Verification items for the finished model (mm, model axes). A direction names the side the tool comes from. Coordinates: 2 decimals unless noted, no trailing zeros. Write each loop counter-clockwise with the first axis right and the second up, starting at its lowest first coordinate (ties: lowest second). Pieces come first, ordered by that corner, then holes.
```python
from build123d import *

# Parameters (mm, degrees)
F0_W          = 30
F0_H          = 30
F1_DEPTH      = 865
F2_W          = 30
F2_H          = 30
F3_DEPTH      = 257.5
F3_DEPTH_BACK = 257.5
F4_W          = 30
F4_H          = 30
F5_DEPTH      = 215
F5_DEPTH_BACK = 215
F6_W          = 480
F6_H          = 30
F7_DEPTH      = 1.5
F8_W          = 480
F8_H          = 1.5
F9_DEPTH      = 28.5
F10_R         = 5


with BuildPart() as f1:
    # F0 (on Top) → F1 (new body)
    with BuildSketch(Plane.XY):
        with Locations((-272.5, 230)):
            Rectangle(F0_W, F0_H)
        with Locations((272.5, 230)):
            Rectangle(F0_W, F0_H)
        with Locations((272.5, -230)):
            Rectangle(F0_W, F0_H)
        with Locations((-272.5, -230)):
            Rectangle(F0_W, F0_H)
    extrude(amount=F1_DEPTH)

    # F2 (on Right) → F3 (join, two sides)
    with BuildSketch(Plane.YZ) as f3_sk:
        with Locations((-230, 100)):
            Rectangle(F2_W, F2_H)
        with Locations((230, 100)):
            Rectangle(F2_W, F2_H)
        with Locations((-230, 850)):
            Rectangle(F2_W, F2_H)
        with Locations((230, 850)):
            Rectangle(F2_W, F2_H)
    extrude(amount=F3_DEPTH)
    extrude(f3_sk.sketch, amount=-F3_DEPTH_BACK)

    # F4 (on Front) → F5 (join, two sides)
    with BuildSketch(Plane.XZ) as f5_sk:
        with Locations((-272.5, 850)):
            Rectangle(F4_W, F4_H)
        with Locations((272.5, 850)):
            Rectangle(F4_W, F4_H)
    extrude(amount=F5_DEPTH)
    extrude(f5_sk.sketch, amount=-F5_DEPTH_BACK)



with BuildPart() as f7:
    # F6 (on face) → F7 (new body)
    with BuildSketch(Plane.YZ.offset(-257.5)):
        with Locations((0, 130)):
            Rectangle(F6_W, F6_H)
        with Locations((0, 300)):
            Rectangle(F6_W, F6_H)
        with Locations((0, 470)):
            Rectangle(F6_W, F6_H)
        with Locations((0, 640)):
            Rectangle(F6_W, F6_H)
    extrude(amount=F7_DEPTH)


with BuildPart() as f1_1:
    add(f1.part)

    add(f7.part)  # F9 merges F7
    # F8 (on face) → F9 (join)
    with BuildSketch(Plane.YZ.offset(-256)):
        with Locations((0, 115.75)):
            Rectangle(F8_W, F8_H)
        with Locations((0, 285.75)):
            Rectangle(F8_W, F8_H)
        with Locations((0, 455.75)):
            Rectangle(F8_W, F8_H)
        with Locations((0, 625.75)):
            Rectangle(F8_W, F8_H)
    extrude(amount=F9_DEPTH)

    # F10
    f10_edges = [f1_1.edges().sort_by_distance(p)[0] for p in [
        (-256.75, -240, 145),
        (-256.75, 240, 145),
        (-227.5, 240, 115.75),
        (-227.5, -240, 115.75),
        (-256.75, -240, 315),
        (-227.5, -240, 285.75),
        (-227.5, -240, 455.75),
        (-256.75, -240, 485),
        (-227.5, -240, 625.75),
        (-256.75, -240, 655),
        (-256.75, 240, 655),
        (-227.5, 240, 625.75),
        (-227.5, 240, 455.75),
        (-256.75, 240, 485),
        (-227.5, 240, 285.75),
        (-256.75, 240, 315),
    ]]
    fillet(f10_edges, radius=F10_R)

    # F11: F1 across plane


with BuildPart() as f1_2:
    add(f1_1.part)
    add(f1_1.part.mirror(Plane.YZ))


solid = f1_2.part
```
1. Material ranges on L1, parallel to Z at x = -253.5, y = 135.5; L2, parallel to Z at x = -235.5, y = -224; L3, parallel to X at y = 211, z = 633.5, recorded low to high.
2. Tool access check on faces 4 (the flat face through (272, -3, 835)), 5 (the flat face through (-251, -240, 286)), 6 (the flat face through (-257.5, -3, 300)), 7 (the flat face through (-257.5, 230, 42)), 8 (the flat face through (-256, -3, 471)). Record the directions out of +Z, -Z, +X, -X, +Y, -Y that give a thin tool (end or side, any length) a straight path to the whole face; none if there is none.
3. Sectioned sample at A-A, the plane x = -62. Record the boundary of the cut face in (y, z), and give its area (3 significant figures).
4. Gauge pin test, flat ends, axial feed: P1, Ø14, axis at y = -6.5, z = 133.5, coming from the +X side; P2, Ø1.6, axis at x = 256.5, y = -40.5, coming from the +Z side; P3, Ø8.5, axis at x = -238.5, y = -100.5, coming from the +Z side; P4, Ø20, axis at x = 251, z = 464.5, coming from the -Y side. Record the tip position at first contact, or that the pin passes through.
5. Sectioned sample at C-C, the plane x = -244. Give the number of separate pieces and of enclosed holes in the cut face, and give its area (3 significant figures).
6. Sectioned sample at B-B, the plane z = 504. Record the boundary of the cut face in (x, y).
7. Draft check along Z on faces 1 (the flat face through (-243, -3, 115)), 2 (the flat face through (-257.5, -230, 42)), 3 (the flat face through (-4, -230, 835)). Enter one of: pulls with the +Z half, pulls with the -Z half, needs draft (parallel to the pull), parting line crosses it, or undercut.
Outcome:
1. L1: z = 115 to 116.5, 285 to 286.5, 455 to 456.5, 625 to 626.5
1. L2: z = 85 to 116.5, 285 to 286.5, 455 to 456.5, 625 to 626.5, 835 to 865
1. L3: x = -257.5 to -256, 256 to 257.5
2. face 4: -Z, +X, -X
2. face 5: -Y
2. face 6: -Z, -X
2. face 7: -Z, +Y, -Y
2. face 8: +Y, -Y
3. outline: (-245, 85) - (-215, 85) - (-215, 115) - (-245, 115) - close; (-245, 835) - (-215, 835) - (-215, 865) - (-245, 865) - close; (215, 85) - (245, 85) - (245, 115) - (215, 115) - close; (215, 835) - (245, 835) - (245, 865) - (215, 865) - close
3. area: 3,600 mm2
4. P1: stops at x = 257.5
4. P2: stops at z = 655
4. P3: stops at z = 626.5
4. P4: stops at y = -245
5. separate pieces: 6
5. enclosed holes: 0
5. area: 6,480 mm2
6. outline: (-287.5, -245) - (-257.5, -245) - (-257.5, -215) - (-287.5, -215) - close; (-287.5, 215) - (-257.5, 215) - (-257.5, 245) - (-287.5, 245) - close; (257.5, -245) - (287.5, -245) - (287.5, -215) - (257.5, -215) - close; (257.5, 215) - (287.5, 215) - (287.5, 245) - (257.5, 245) - close
7. face 1: pulls with the -Z half
7. face 2: needs draft
7. face 3: undercut
